Input: part model. Units: mm. Frame: model coordinates. Face numbers are marked on the shaded views. A direction names the side the tool comes from. Coordinates: 2 decimals unless noted, no trailing zeros. Write each loop counter-clockwise with the first axis right and the second up, starting at its lowest first coordinate (ties: lowest second). Pieces come first, ordered by that corner, then holes.
1) Line query: L1, parallel to X at y = 2.25, z = 1.25; L2, parallel to Y at x = 5.5, z = 9.75; L3, parallel to Y at x = 15.5, z = 3.5. Output: solid intervals per line, ascending.
2) Section query B-B (y = 4.5). Output: boundary loops of the cut face in (x, z), then the cut area to 3 significant figures.
3) Pin query (flat end, axial travel): pin 1 Ø5.5 at (y, z) = (3.5, 8) entering from -X; pin 2 Ø1.5 at (x, z) = (6.5, 3.5) entering from -Y. Return the tip coordinate at first contact, or that it passes through.
4) Section query A-A (z = 5.5). Output: boundary loops of the cut face in (x, y).
5) Set-up query: the marked faces 1 and 2. Return all of +Z, -Z, +X, -X, +Y, -Y with unobstructed straight access to the full face (end or side cutting, diameter ignored); none if empty.
6) Section query C-C (x = 6.75). Output: boundary loops of the cut face in (y, z).
from build123d import *

# Parameters (mm, degrees)
F0_W     = 16.4
F0_H     = 19.2
F1_DEPTH = 11.3
F2_W     = 11.3
F2_H     = 11.3
F3_DEPTH = 25
F4_R     = 2
F5_R     = 1


with BuildPart() as f1:
    # F0 (on Top) → F1 (new body)
    with BuildSketch(Plane.XY):
        with Locations((8.2, 9.6)):
            Rectangle(F0_W, F0_H)
    extrude(amount=F1_DEPTH)

    # F2 (on face) → F3 (cut)
    with BuildSketch(Plane.XY.offset(11.3)):
        with Locations((5.65, 5.65)):
            Rectangle(F2_W, F2_H)
    extrude(amount=-F3_DEPTH, mode=Mode.SUBTRACT)

    # F4
    f4_edges = [f1.edges().sort_by_distance(p)[0] for p in [
        (13.85, 0, 0),
        (0, 15.25, 0),
    ]]
    fillet(f4_edges, radius=F4_R)

    # F5
    f5_edges = [f1.edges().sort_by_distance(p)[0] for p in [
        (8.2, 19.2, 11.3),
        (16.4, 9.6, 11.3),
        (16.4, 19.2, 5.65),
    ]]
    fillet(f5_edges, radius=F5_R)


solid = f1.part
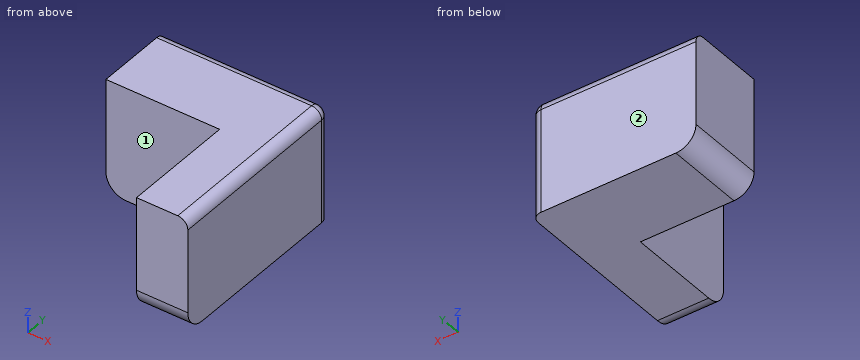
Answer:
1. L1: x = 11.3 to 16.4
1. L2: y = 11.3 to 19.2
1. L3: y = 0 to 19.19
2. outline: (11.3, 0) - (16.4, 0) - (16.4, 10.3) arc R1 ccw to (15.4, 11.3) - (11.3, 11.3) - close
2. area: 57.4 mm2
3. pin 1: stops at x = 11.3
3. pin 2: stops at y = 11.3
4. outline: (0, 11.3) - (11.3, 11.3) - (11.3, 0) - (16.4, 0) - (16.4, 18.2) arc R1 ccw to (15.4, 19.2) - (0, 19.2) - close
5. face 1: +Z, -Z, -X, -Y
5. face 2: +Z, -Z, +X, -X, +Y
6. outline: (11.3, 0) - (19.2, 0) - (19.2, 10.3) arc R1 ccw to (18.2, 11.3) - (11.3, 11.3) - close
